Geometry check sheet. Reference: the model listing, model coordinates, mm. A direction names the side the tool comes from. Give positions to 0.01 mm unless a question says otherwise; leave off trailing zeros. Loops run counter-clockwise (first coordinate to the right, second up) from the corner with the lowest first, then second, coordinate; pieces in that order, holes last. Notation, with made-up numbers: (-4, 28) -> (42, 28) arc R16 ccw to (42, 58) -> close; hole circle Ø10 at (-19, 50). An arc over 180 degrees is marked (long way). One line per item, written item: value. Start each with the question number.
(1) Gauge pin test, flat ends, axial feed: pin 1 Ø1.2 at (y, z) = (24.94, 9.86) entering from +X; pin 2 Ø24 at (x, y) = (34, 22) entering from +Z; pin 3 Ø1 at (x, y) = (44, 24.5) entering from -Z; pin 4 Ø1 at (x, z) = (48.5, 6) entering from -Y. Record the tip position at first contact, or that the pin passes through.
(2) Tool access check on faces 5 (the face through (52.465, 31.635, 9.675)), 6 (the face through (25, 25, 20)), 7 (the face through (25, 25, 0)), 8 (the face through (56.01, 41.14, 14.17)). Record the directions out of +Z, -Z, +X, -X, +Y, -Y that give a thin tool (end or side, any length) a straight path to the whole face; none if there is none.
(3) Draft check along X on faces 1 (the face through (50, 25, 10)), 2 (the face through (56.014, 27.234, 5.166)), 3 (the face through (55, 34, 7)), 4 (the face through (57, 34, 10)). Enter one of: pulls with the +X half, pulls with the -X half, needs draft (parallel to the pull), parting line crosses it, or undercut.
(4) Sectioned sample at A-A, the plane y = 12.5. Record the cut outline in (x, z).
(5) Scan lines: line 1 along X through (y, z) = (15, 7); line 2 along Z through (x, y) = (33.5, 35.5); line 3 along X through (y, z) = (39, -1). Record each from-to range of solid material in increasing order. Write a range as from..to.
from build123d import *

# Parameters (mm, degrees)
SKETCH1_W           = 50
SKETCH1_H           = 50
BOSS_EXTRUDE1_DEPTH = 20
SKETCH2_R           = 2.5
BOSS_EXTRUDE2_DEPTH = 5
SKETCH3_R           = 12.5
BOSS_EXTRUDE3_DEPTH = 2
FILLET1_R           = 1
CIRPATTERN1_COUNT   = 12


with BuildPart() as part:
    # Sketch1 → Boss-Extrude1 (new body)
    with BuildSketch(Plane.XY):
        with Locations((25, 25)):
            Rectangle(SKETCH1_W, SKETCH1_H)
    extrude(amount=BOSS_EXTRUDE1_DEPTH)

    # Sketch2 → Boss-Extrude2 (add)
    with BuildSketch(Plane(origin=(50, 0, 0), x_dir=(0, 0, -1), z_dir=(1, 0, 0))):
        with Locations(Location((-10, 34.113262312, 0), (0, 0, 180))):
            Circle(SKETCH2_R)
    extrude(amount=BOSS_EXTRUDE2_DEPTH)

    # Sketch3 → Boss-Extrude3 (add)
    with BuildSketch(Plane(origin=(55, 0, 0), x_dir=(0, 0, -1), z_dir=(1, 0, 0))):
        with Locations((-10, 34.113262312)):
            Circle(SKETCH3_R)
    extrude(amount=BOSS_EXTRUDE3_DEPTH)

    # Fillet1
    fillet1_edges = [part.edges().sort_by_distance(p)[0] for p in [
        (50, 25, 20),
        (25, 50, 20),
        (0, 25, 20),
        (25, 50, 0),
        (50, 25, 0),
        (25, 0, 0),
        (0, 25, 0),
        (25, 0, 20),
        (0, 50, 10),
        (50, 50, 10),
        (50, 0, 10),
        (0, 0, 10),
    ]]
    fillet(fillet1_edges, radius=FILLET1_R)

    # Sketch4 → Ø2.0mm Dowel Hole1 (revolve, cut)
    with BuildSketch(Plane(origin=(57, 34.25166224, 0.83161613), x_dir=(0, 0, -1), z_dir=(0, 1, 0))):
        Polygon((0, 0), (0, 2.600860619), (1, 2), (1, 0), align=None)
    f_2_0mm_dowel_hole1 = revolve(axis=Axis((63.35, 34.25166224, 0.83161613), (-1, 0, 0)), mode=Mode.SUBTRACT)

    # CirPattern1: Ø2.0mm Dowel Hole1 ×12 about axis
    cirpattern1_axis = Axis((0, 34.113262312, 10), (1, 0, 0))
    for i in range(1, CIRPATTERN1_COUNT):
        add(f_2_0mm_dowel_hole1.rotate(cirpattern1_axis, i * 360 / CIRPATTERN1_COUNT), mode=Mode.SUBTRACT)


solid = part.part
Calculated:
1. pin 1: stops at x = 50
1. pin 2: stops at z = 20
1. pin 3: stops at z = 0
1. pin 4: stops at y = 0
2. face 5: none
2. face 6: +Z, -X, +Y, -Y
2. face 7: -Z, -X, +Y, -Y
2. face 8: +X
3. face 1: undercut
3. face 2: needs draft
3. face 3: undercut
3. face 4: pulls with the +X half
4. outline: (0, 1) arc R1 ccw to (1, 0) -> (49, 0) arc R1 ccw to (50, 1) -> (50, 19) arc R1 ccw to (49, 20) -> (1, 20) arc R1 ccw to (0, 19) -> close
5. line 1: x = 0..50
5. line 2: z = 0..20
5. line 3: x = 55..57
